```python
from build123d import *

# Parameters (mm, degrees)
SKETCH1_R           = 6.25
BOSS_EXTRUDE1_DEPTH = 7


with BuildPart() as part:
    # Sketch1 → Boss-Extrude1 (new body)
    with BuildSketch(Plane(origin=(0, 0, 0), x_dir=(1, 0, 0), z_dir=(0, 1, 0))):
        with BuildLine():
            Line((72.34, -63.405178012), (38.75, -96.995178012))
            Line((38.75, -96.995178012), (38.75, -111.995178012))
            Line((38.75, -111.995178012), (87.34, -111.995178012))
            Line((87.34, -111.995178012), (87.34, -94.896256746))
            Line((87.34, -94.896256746), (82.922661505, -99.760117279))
            ThreePointArc((82.922661505, -99.760117279), (79.206389469, -106.17642477), (79.948751144, -98.798852079))
            Line((79.948751144, -98.798852079), (87.34, -90.296256746))
            Line((87.34, -90.296256746), (87.34, -63.405178012))
            Line((87.34, -63.405178012), (72.34, -63.405178012))
        make_face()
        with Locations(Location((65.34, -89.995178012, 0), (0, 0, 270))):
            Circle(SKETCH1_R, mode=Mode.SUBTRACT)
    extrude(amount=BOSS_EXTRUDE1_DEPTH)


solid = part.part
```
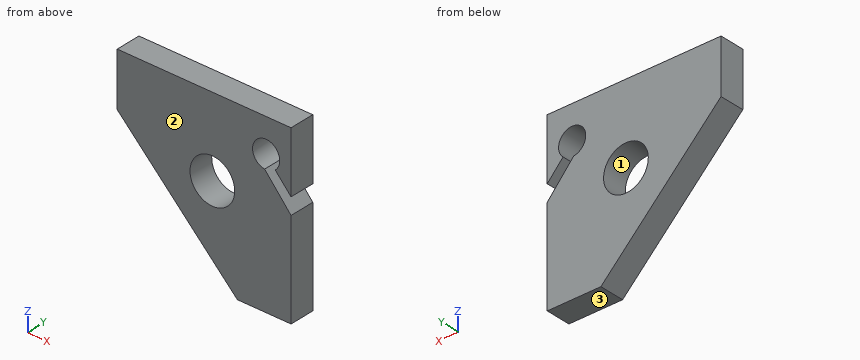
Check sheet for the modelled part. Datum: model origin and axes. Units: mm. Face numbers are marked on the shaded views. Give positions to 0.01 mm unless a question says otherwise; leave off trailing zeros. Order: outer loops, then holes, each group sorted by start corner. A loop starts at its lowest first (then second) coordinate and runs counter-clockwise, first axis right, second up. Notation, with made-up numbers: M 15,-20 L 53,-20 A7 cw 53,-15 Z; hole C -18,-4.75 d7. An arc over 180 degrees is marked long. Answer in a Markdown table with one row per item. Add a question column.
Q1. Thickness scan on L1, parallel to X at y = 5.25, z = 95.5; L2, parallel to Z at x = 63.5, y = 3; L3, parallel to Z at x = 79, y = 5.75. Record the ranges inside material, lowest first.
Q2. Sectioned sample at D-D, the plane z = 72. Record the boundary of the cut face in (x, y).
Q3. Sectioned sample at A-A, the plane y = 6.25. Record the boundary of the cut face in (x, z).
Q4. Release check for a two-part mould opening along Z. For the marked faces 1, 2 and 3 record: released by +Z, released by -Z, zero draft, split by the parting line, or undercut.
Q5. Sectioned sample at C-C, the plane z = 89.5. Record the boundary of the cut face in (x, y).
Q6. Sectioned sample at B-B, the plane x = 65.34. Record the boundary of the cut face in (y, z), and give its area (3 significant figures).
Verdict:
| question | item | result |
|---|---|---|
| 1 | L1 | 40.25 to 62.38, 68.3 to 82.82, 86.79 to 87.34 |
| 1 | L2 | 72.25 to 84.02, 95.97 to 112 |
| 1 | L3 | 63.41 to 99.03, 106.1 to 112 |
| 2 | outline | M 63.75,0 L 87.34,0 L 87.34,7 L 63.75,7 Z |
| 3 | outline | M 38.75,97 L 72.34,63.41 L 87.34,63.41 L 87.34,90.3 L 79.95,98.8 A3.79 cw long 82.92,99.76 L 87.34,94.9 L 87.34,112 L 38.75,112 Z; hole C 65.34,90 d12.5 |
| 4 | face 1 | undercut |
| 4 | face 2 | zero draft |
| 4 | face 3 | released by -Z |
| 5 | outline | M 46.25,0 L 59.11,0 L 59.11,7 L 46.25,7 Z; M 71.57,0 L 87.34,0 L 87.34,7 L 71.57,7 Z |
| 6 | outline | M 0,70.41 L 7,70.41 L 7,83.75 L 0,83.75 Z; M 0,96.25 L 7,96.25 L 7,112 L 0,112 Z |
| 6 | area | 204 mm² |
